Read the model definition and answer for the solid it produces. Units are mm, in the model's axes. Face numbers are marked on the shaded views. A direction names the side the tool comes from. Coordinates: 2 decimals unless noted, no trailing zeros. Write each loop counter-clockwise with the first axis right and the second up, starting at its lowest first coordinate (ties: lowest second). Pieces come first, ordered by that corner, then holes. Notation, with made-up numbers: (-5, -29) -> (45, -29) arc R16 ccw to (45, -10) -> close; hole circle Ø3 at (15, 47.5). An arc over 180 degrees is marked (long way). Write item = value, one per line. Start each with the question number.
1) Flat-ended cylindrical pins translate along their axes: pin 1 Ø1.8 at (y, z) = (3.5, 5.5) entering from +X; pin 2 Ø1.8 at (y, z) = (4, 5.5) entering from -X; pin 3 Ø10 at (x, z) = (57.5, 11.5) entering from -Y. Find the tip coordinate at first contact, or state that the pin passes through.
2) Section B-B (z = 6.25) is taken. Determine the outline of the cut face in (x, y) (3 decimals), plus the area to 3 significant figures.
3) For a pull along X with two mould halves and no side action, classify the marked faces 3 and 4 as released by +X, released by -X, zero draft, split by the parting line, or undercut.
4) A tool of negligible diameter and unlimited length cuts with its end or side. For the marked faces 1 and 2, from which of +Z, -Z, +X, -X, +Y, -Y can it reach the whole face along a straight path? Write none if from no direction.
5) Section A-A (x = -41) is taken. Determine the outline of the cut face in (y, z).
6) Find the intervals of material crossed by line 1 along Y through (x, z) = (-41, 1.85); line 2 along Z through (x, y) = (44, -8.75); line 3 along Z through (x, y) = (-91, 1), in increasing order. Write a range as from..to.
7) Section D-D (z = 15) is taken. Determine the outline of the cut face in (x, y).
8) Section C-C (x = -85) is taken. Determine the outline of the cut face in (y, z).
from build123d import *

# Parameters (mm, degrees)
SKETCH1_R           = 5
BOSS_EXTRUDE1_DEPTH = 3
BOSS_EXTRUDE2_DEPTH = 6
CHAMFER1_START      = -106
CHAMFER1_DEPTH      = 45
CHAMFER1_START_2    = -22.5
CHAMFER1_2_DEPTH    = 45
CHAMFER1_START_3    = 61
CHAMFER1_3_DEPTH    = 45
CHAMFER1_START_4    = -4
CHAMFER1_4_DEPTH    = 9.159204648
CHAMFER1_START_5    = 3
CHAMFER1_5_DEPTH    = 10
FILLET1_R           = 10


with BuildPart() as part:
    # Sketch1 → Boss-Extrude1 (new body)
    with BuildSketch(Plane.XY):
        with BuildLine():
            Line((-106, -10), (106, -10))
            Line((106, -10), (106, 0))
            ThreePointArc((106, 0), (103.071067812, 7.071067812), (96, 10))
            Line((96, 10), (-96, 10))
            ThreePointArc((-96, 10), (-103.071067812, 7.071067812), (-106, 0))
            Line((-106, 0), (-106, -10))
        make_face()
        with Locations((-41, 0)):
            Circle(SKETCH1_R, mode=Mode.SUBTRACT)
        with Locations((41, 0)):
            Circle(SKETCH1_R, mode=Mode.SUBTRACT)
    extrude(amount=BOSS_EXTRUDE1_DEPTH)

    # Sketch2 → Boss-Extrude2 (add)
    with BuildSketch(Plane.XZ.offset(10)):
        with BuildLine():
            Line((-106, 0), (-61, 0))
            Line((-61, 0), (-61, 12))
            ThreePointArc((-61, 12), (-63.928932188, 19.071067812), (-71, 22))
            Line((-71, 22), (-96, 22))
            ThreePointArc((-96, 22), (-103.071067812, 19.071067812), (-106, 12))
            Line((-106, 12), (-106, 0))
        make_face()
        with BuildLine():
            Line((106, 0), (61, 0))
            Line((61, 0), (61, 12))
            ThreePointArc((61, 12), (63.928932188, 19.071067812), (71, 22))
            Line((71, 22), (96, 22))
            ThreePointArc((96, 22), (103.071067812, 19.071067812), (106, 12))
            Line((106, 12), (106, 0))
        make_face()
        with BuildLine():
            Line((-22.5, 0), (22.5, 0))
            Line((22.5, 0), (22.5, 12))
            ThreePointArc((22.5, 12), (19.571067812, 19.071067812), (12.5, 22))
            Line((12.5, 22), (-12.5, 22))
            ThreePointArc((-12.5, 22), (-19.571067812, 19.071067812), (-22.5, 12))
            Line((-22.5, 12), (-22.5, 0))
        make_face()
    extrude(amount=-BOSS_EXTRUDE2_DEPTH)

    # Chamfer1: read off the stored shape, not the designer's step
    # Chamfer1 outline → Chamfer1 (add)
    with BuildSketch(Plane.YZ.offset(CHAMFER1_START)):
        Polygon((6, 3), (-3.5, 22), (-4, 22), (-4, 3), align=None)
    extrude(amount=CHAMFER1_DEPTH)

    # Chamfer1 2 outline → Chamfer1 2 (add)
    with BuildSketch(Plane.YZ.offset(CHAMFER1_START_2)):
        Polygon((6, 3), (-3.5, 22), (-4, 22), (-4, 3), align=None)
    extrude(amount=CHAMFER1_2_DEPTH)

    # Chamfer1 3 outline → Chamfer1 3 (add)
    with BuildSketch(Plane.YZ.offset(CHAMFER1_START_3)):
        Polygon((6, 3), (-3.5, 22), (-4, 22), (-4, 3), align=None)
    extrude(amount=CHAMFER1_3_DEPTH)

    # Chamfer1 4 outline → Chamfer1 4 (cut)
    with BuildSketch(Plane(origin=(0, 0, 0), x_dir=(1, 0, 0), z_dir=(0, 1, 0)).offset(CHAMFER1_START_4)):
        with BuildLine():
            Line((-106, -22), (-96, -22))
            ThreePointArc((-96, -22), (-103.071067812, -19.071067812), (-106, -12))
            Line((-106, -12), (-106, -22))
        make_face()
        with BuildLine():
            ThreePointArc((-61, -12), (-63.928932188, -19.071067812), (-71, -22))
            Line((-71, -22), (-61, -22))
            Line((-61, -22), (-61, -12))
        make_face()
        with BuildLine():
            Line((61, -22), (71, -22))
            ThreePointArc((71, -22), (63.928932188, -19.071067812), (61, -12))
            Line((61, -12), (61, -22))
        make_face()
        with BuildLine():
            ThreePointArc((106, -12), (103.071067812, -19.071067812), (96, -22))
            Line((96, -22), (106, -22))
            Line((106, -22), (106, -12))
        make_face()
        with BuildLine():
            Line((-22.5, -22), (-12.5, -22))
            ThreePointArc((-12.5, -22), (-19.571067812, -19.071067812), (-22.5, -12))
            Line((-22.5, -12), (-22.5, -22))
        make_face()
        with BuildLine():
            ThreePointArc((22.5, -12), (19.571067812, -19.071067812), (12.5, -22))
            Line((12.5, -22), (22.5, -22))
            Line((22.5, -22), (22.5, -12))
        make_face()
    extrude(amount=CHAMFER1_4_DEPTH, mode=Mode.SUBTRACT)

    # Chamfer1 5 outline → Chamfer1 5 (cut)
    with BuildSketch(Plane.XY.offset(CHAMFER1_START_5)):
        with BuildLine():
            Line((106, 7), (103.141428429, 7))
            ThreePointArc((103.141428429, 7), (105.257815193, 3.780589618), (106, 0))
            Line((106, 0), (106, 7))
        make_face()
        with BuildLine():
            ThreePointArc((-106, 0), (-105.257815193, 3.780589618), (-103.141428429, 7))
            Line((-103.141428429, 7), (-106, 7))
            Line((-106, 7), (-106, 0))
        make_face()
    extrude(amount=CHAMFER1_5_DEPTH, mode=Mode.SUBTRACT)

    # Fillet1
    # the kernel refuses this fillet: 10 mm, written as the material it takes off along each edge
    with BuildSketch(Plane(origin=(-106, -10, -25), x_dir=(1, 0, 0), z_dir=(0, 0, 1))) as fillet1_piece_1:
        with BuildLine():
            CenterArc((FILLET1_R, FILLET1_R), FILLET1_R, 180, 90)
            Line((0, FILLET1_R), (0, 0))
            Line((0, 0), (FILLET1_R, 0))
        make_face()
    extrude(amount=62, mode=Mode.SUBTRACT)
    with BuildSketch(Plane(origin=(-61, -10, 3), x_dir=(-1, 0, 0), z_dir=(0, 0, 1)), Plane(origin=(61, -10, 3), x_dir=(0, 1, 0), z_dir=(0, 0, 1)), Plane(origin=(-22.5, -10, 37), x_dir=(1, 0, 0), z_dir=(0, 0, -1)), Plane(origin=(22.5, -10, 3), x_dir=(-1, 0, 0), z_dir=(0, 0, 1))) as fillet1_piece_2:
        with BuildLine():
            CenterArc((FILLET1_R, -FILLET1_R), FILLET1_R, 90, 90)
            Line((0, -FILLET1_R), (0, 0))
            Line((0, 0), (FILLET1_R, 0))
        make_face()
    extrude(amount=34, mode=Mode.SUBTRACT)
    with BuildSketch(Plane(origin=(106, -10, 37), x_dir=(0, 1, 0), z_dir=(0, 0, -1))) as fillet1_piece_3:
        with BuildLine():
            CenterArc((FILLET1_R, -FILLET1_R), FILLET1_R, 90, 90)
            Line((0, -FILLET1_R), (0, 0))
            Line((0, 0), (FILLET1_R, 0))
        make_face()
    extrude(amount=62, mode=Mode.SUBTRACT)


solid = part.part
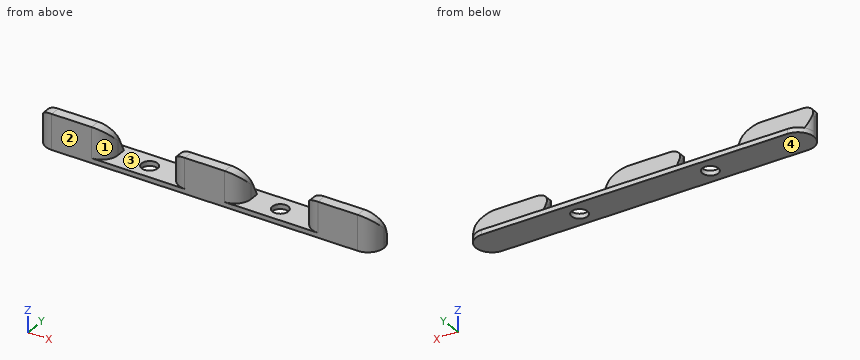
Answer key:
q1.pin_1 = 105.66
q1.pin_2 = -105.51
q1.pin_3 = -5.27
q2.outline = (-104.992, 4.375) arc R10 ccw to (-96, -10) -> (-71, -10) arc R10 ccw to (-61, 0) -> (-61, 4.375) -> close; (-22.5, 0) arc R10 ccw to (-12.5, -10) -> (12.5, -10) arc R10 ccw to (22.5, 0) -> (22.5, 4.375) -> (-22.5, 4.375) -> close; (61, 0) arc R10 ccw to (71, -10) -> (96, -10) arc R10 ccw to (104.992, 4.375) -> (61, 4.375) -> close
q2.area = 1,810 mm^2
q3.face_3 = undercut
q3.face_4 = zero draft
q4.face_1 = +Z, -Y
q4.face_2 = +Z, -Z, +X, -X, -Y
q5.outline = (-10, 0) -> (-5, 0) -> (-5, 3) -> (-10, 3) -> close; (5, 0) -> (10, 0) -> (10, 3) -> (5, 3) -> close
q6.line_1 = -10..-5, 5..10
q6.line_2 = 0..3
q6.line_3 = 0..13
q7.outline = (-105.54, -3) arc R10 ccw to (-96, -10) -> (-71, -10) arc R10 ccw to (-61.46, -3) -> (-61.46, 0) -> (-105.54, 0) -> close; (-22.04, -3) arc R10 ccw to (-12.5, -10) -> (12.5, -10) arc R10 ccw to (22.04, -3) -> (22.04, 0) -> (-22.04, 0) -> close; (61.46, -3) arc R10 ccw to (71, -10) -> (96, -10) arc R10 ccw to (105.54, -3) -> (105.54, 0) -> (61.46, 0) -> close
q8.outline = (-10, 0) -> (10, 0) -> (10, 3) -> (6, 3) -> (-3.5, 22) -> (-10, 22) -> close
